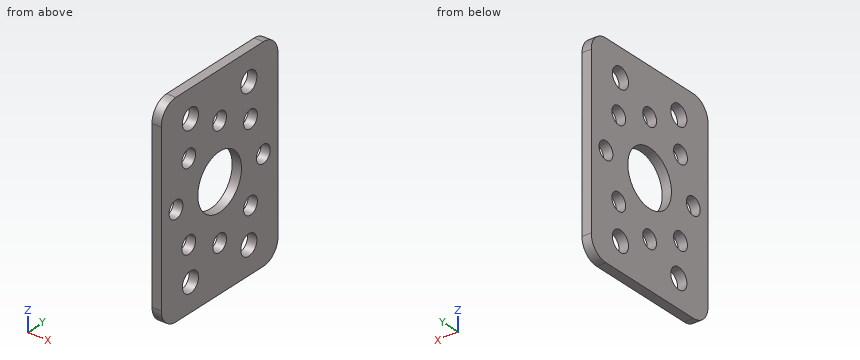
Autodesk Inventor part; units mm, degrees
ref_plane "YZ Plane" through (0, 0, 0) normal (1, 0, 0) x (0, 1, 0)
ref_plane "XZ Plane" through (0, 0, 0) normal (0, 1, 0) x (-1, 0, 0)
ref_plane "XY Plane" through (0, 0, 0) normal (0, 0, 1) x (1, 0, 0)
sketch "Sketch1" plane through (0, 0, 0) normal (1, 0, 0) x (0, 1, 0)
  circle A0 centre (0, 0) radius 4.75
  line L0 (0, 0) -> (0, -12.7) construction
  line L1 (0, -12.7) -> (6.35, -12.7) construction
  circle A1 centre (6.35, -12.7) radius 1.7526
  circle A2 centre (-6.35, -12.7) radius 1.7526
  circle A3 centre (6.35, 12.7) radius 1.7526
  circle A4 centre (-6.35, 12.7) radius 1.7526
  line L2 (12.7, 17.4625) -> (-12.7, 17.4625)
  line L3 (-12.7, 17.4625) -> (-12.7, -17.4625)
  line L4 (-12.7, -17.4625) -> (12.7, -17.4625)
  line L5 (12.7, -17.4625) -> (12.7, 17.4625)
  line L6 (12.7, 17.4625) -> (-12.7, -17.4625) construction
  line L7 (-12.7, 17.4625) -> (12.7, -17.4625) construction
  circle A5 centre (9.5, 0) radius 1.5 construction
  line L8 (0, 0) -> (9.5, 0) construction
  circle A6 centre (0, 0) radius 9.5 construction
  circle A7 centre (6.7175, 6.7175) radius 1.5
  line L9 (6.7175, 6.7175) -> (0, 0) construction
  circle A8 centre (0, 9.5) radius 1.5
  circle A9 centre (-6.7175, 6.7175) radius 1.5
  circle A10 centre (-9.5, 0) radius 1.5
  circle A11 centre (-6.7175, -6.7175) radius 1.5
  circle A12 centre (0, -9.5) radius 1.5
  circle A13 centre (6.7175, -6.7175) radius 1.5
  circle A14 centre (9.5, 0) radius 1.5
  dimension "d0" = 9.5
  dimension "d1" = 12.7
  dimension "d2" = 6.35
  dimension "d3" = 3.5052
  dimension "d6" = 12.7
  dimension "d9" = 25.4
  dimension "d12" = 25.4
  dimension "d13" = 34.925
  dimension "d14" = 3
  dimension "d15" = 9.5
  dimension "d23" = 3
  dimension "d24" = 45
  dimension "d27" = 360
extrude "Extrusion1" add sketch "Sketch1" along normal blind 1.5875
fillet "Fillet1" radius 3.175 4 edges at (0.7937, 12.7, 17.4625) (0.7937, -12.7, 17.4625) (0.7937, 12.7, -17.4625) (0.7937, -12.7, -17.4625)
equation "\"d9\" = 2 * d1"
equation "\"d23\" = d14"
properties part number "Motor Plates" material "Aluminum 6061"
Model file for the job. Use its own axes, mm. Coordinates: 2 decimals unless noted, no trailing zeros. Write each loop counter-clockwise with the first axis right and the second up, starting at its lowest first coordinate (ties: lowest second). Pieces come first, ordered by that corner, then holes. Notation, with made-up numbers: (82, 8) - (91, 8) arc R16 cw to (91, 38) - close; hole circle Ø8 at (-30.75, -39). An arc over 180 degrees is marked (long way). Use a Markdown table: item, result. Add a question column.
Item 1: Band-saw the part on D-D, the plane z = -3.5. Write the cut outline in (x, y).
Item 2: Band-saw the part on C-C, the plane z = 12.7. Write the cut outline in (x, y).
Item 3: Band-saw the part on B-B, the plane y = 0. Write the cut outline in (x, z).
Item 4: Drill centre lines: line 1 along Z through (x, y) = (0.55, 0); line 2 along Y through (x, z) = (0.25, 13.5); line 3 along Y through (x, z) = (1.5, 11.5). Where is each one in solid material? Low to high.
Item 5: Drop a flat-ended pin along its axis: pin 1 (2.5 mm diameter, centred on y = 0, z = 9.5, fed in from +X). Give the stop position or say it passes through.
Item 6: Band-saw the part on A-A, the plane z = 0. Write the cut outline in (x, y), and give its area (3 significant figures).
A:
| question | item | result |
|---|---|---|
| 1 | outline | (0, -12.7) - (1.59, -12.7) - (1.59, -3.21) - (0, -3.21) - close; (0, 3.21) - (1.59, 3.21) - (1.59, 12.7) - (0, 12.7) - close |
| 2 | outline | (0, -12.7) - (1.59, -12.7) - (1.59, -8.1) - (0, -8.1) - close; (0, -4.6) - (1.59, -4.6) - (1.59, 4.6) - (0, 4.6) - close; (0, 8.1) - (1.59, 8.1) - (1.59, 12.7) - (0, 12.7) - close |
| 3 | outline | (0, -17.46) - (1.59, -17.46) - (1.59, -11) - (0, -11) - close; (0, -8) - (1.59, -8) - (1.59, -4.75) - (0, -4.75) - close; (0, 4.75) - (1.59, 4.75) - (1.59, 8) - (0, 8) - close; (0, 11) - (1.59, 11) - (1.59, 17.46) - (0, 17.46) - close |
| 4 | line 1 | z = -17.46 to -11, -8 to -4.75, 4.75 to 8, 11 to 17.46 |
| 4 | line 2 | y = -12.7 to -7.91, -4.79 to 4.79, 7.91 to 12.7 |
| 4 | line 3 | y = -12.7 to -7.63, -5.07 to 5.07, 7.63 to 12.7 |
| 5 | pin 1 | passes through |
| 6 | outline | (0, -12.7) - (1.59, -12.7) - (1.59, -11) - (0, -11) - close; (0, -8) - (1.59, -8) - (1.59, -4.75) - (0, -4.75) - close; (0, 4.75) - (1.59, 4.75) - (1.59, 8) - (0, 8) - close; (0, 11) - (1.59, 11) - (1.59, 12.7) - (0, 12.7) - close |
| 6 | area | 15.7 mm² |
